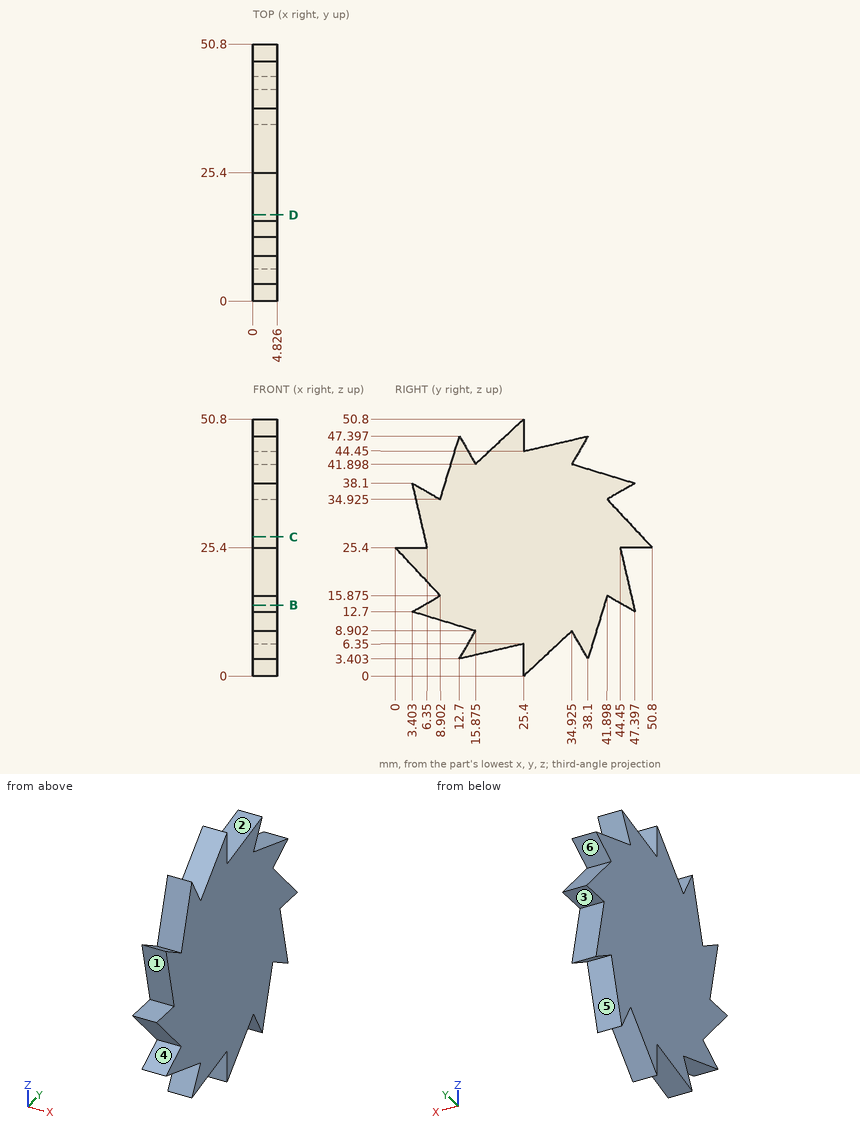
Here's the drawing with two shaded views (mm, measured from the low corner). I have some questions. A direction names the side the tool comes from. Coordinates: 2 decimals unless noted, no trailing zeros. Write each loop counter-clockwise with the first axis right and the second up, starting at its lowest first coordinate (ties: lowest second). Pieces come first, ordered by that corner, then holes. Notation, with made-up numbers: (10.25, 28.5) - (33.25, 28.5) arc R28 cw to (33.25, 49.5) - close; hole circle Ø8 at (50.5, -37.5). An arc over 180 degrees is marked (long way). Return JSON: item names as keys, results as strings.
Q1. Thinking about a two-plate mould opening in Y: for the marked faces 1, 2 and 3, which applies, +Y half, -Y half, draft (parallel to the pull), parting line (faces both ways), or undercut?
Computed values:
{"face 1": "-Y half", "face 2": "undercut", "face 3": "draft"}
Q2. On a 3-axis mill with a long thin cutter (end or side, diameter ignored), from which of +Z, -Z, +X, -X, +Y, -Y can I reach the whole of each face in a straight line? I mean the marked faces 4, 5 and 6. Say none if no direction works.
Computed values:
{"face 4": "+X, -X, -Y", "face 5": "-Z, +X, -X", "face 6": "+X, -X, +Y"}
Q3. If we section it at B-B (z = 14): Please give me the cut outline in (x, y) (1 decimal).
Computed values:
{"outline": "(0, 5.7) - (4.8, 5.7) - (4.8, 41.3) - (0, 41.3) - close; (0, 45.1) - (4.8, 45.1) - (4.8, 47.1) - (0, 47.1) - close"}
Q4. Please list where these lines run through material, in increasing order: L1, parallel to Z at x = 4.25, y = 14 (1 decimal); L2, parallel to Z at x = 2.65, y = 8 (1 decimal); L3, parallel to Z at x = 4.1, y = 33. Write a range as from..to.
Computed values:
{"L1": "z = 3.7..5.7, 9.5..45.1", "L2": "z = 11.3..15.4, 16.8..35.4", "L3": "z = 7.1..46.21"}
Q5. If we section it at D-D (y = 17): Please give me the cut outline in (x, z), then the cut area to 3 significant figures.
Computed values:
{"outline": "(0, 4.4) - (4.83, 4.4) - (4.83, 42.95) - (0, 42.95) - close", "area": "186 mm2"}
Q6. If we section it at C-C (z = 27.5): Please give me the cut outline in (x, y).
Computed values:
{"outline": "(0, 5.86) - (4.83, 5.86) - (4.83, 48.84) - (0, 48.84) - close"}
Q7. I'm going to push flat-ended pins straight in: pin 1 Ø1.4 at (x, z) = (1.5, 47) entering from +Y; pin 2 Ø1.5 at (x, z) = (3, 28) entering from +Y. Where does each tip first touch, or does it pass through?
Computed values:
{"pin 1": "stops at y = 38.1", "pin 2": "stops at y = 49.07"}
